Model file for the job. Use its own axes, mm. Face numbers are marked on the shaded views. A direction names the side the tool comes from. Give positions to 0.01 mm unless a question says otherwise; leave off trailing zeros. Write each loop counter-clockwise with the first axis right and the second up, starting at its lowest first coordinate (ties: lowest second). Pieces come first, ordered by that corner, then holes. Notation, with made-up numbers: (61, 57) - (119, 57) arc R22 cw to (119, 90) - close; hole circle Ø8 at (47.25, 0.25). An arc over 180 degrees is marked (long way). Use CSV: the item, a comma, the result in double quotes.
from build123d import *

# Parameters (mm, degrees)
BOSS_EXTRUDE1_DEPTH     = 80
SHELL1_T                = -2
SKETCH2_W               = 15.034493015
SKETCH2_H               = 76
SKETCH2_W_2             = 15.087666062
BOSS_EXTRUDE2_DEPTH     = 2
CUT_EXTRUDE1_REACH      = 82
CUT_EXTRUDE2_REACH      = 82
SKETCH6_R               = 2
CUT_EXTRUDE6_DEPTH      = 61
LPATTERN1_COUNT         = 4
LPATTERN1_PITCH         = 20
MIRROR1_COPY_1_SKETCH_R = 2
MIRROR1_COPY_1_DEPTH    = 61
MIRROR1_COPY_2_SKETCH_R = 2
MIRROR1_COPY_2_DEPTH    = 61
MIRROR1_COPY_3_SKETCH_R = 2
MIRROR1_COPY_3_DEPTH    = 61


with BuildPart() as part:
    # Sketch1 → Boss-Extrude1 (new body)
    with BuildSketch(Plane.XY):
        with BuildLine():
            Line((-75, 0), (75, 0))
            Line((75, 0), (75, 4))
            Line((75, 4), (59.866518188, 4))
            ThreePointArc((59.866518188, 4), (0, 60), (-59.866518188, 4))
            Line((-59.866518188, 4), (-75, 4))
            Line((-75, 4), (-75, 0))
        make_face()
    extrude(amount=BOSS_EXTRUDE1_DEPTH)

    # Shell1
    shell1_openings = [part.faces().sort_by_distance(p)[0] for p in [
        (0, 0, 40),
    ]]
    offset(amount=SHELL1_T, openings=shell1_openings, kind=Kind.INTERSECTION)

    # Sketch2 → Boss-Extrude2 (add)
    with BuildSketch(Plane.XZ.offset(-2)):
        with Locations((-65.482753492, 40)):
            Rectangle(SKETCH2_W, SKETCH2_H)
        with Locations((65.456166969, 40)):
            Rectangle(SKETCH2_W_2, SKETCH2_H)
    extrude(amount=BOSS_EXTRUDE2_DEPTH)

    # Sketch3 → Cut-Extrude1 (cut, up to next)
    with BuildSketch(Plane.XY.offset(80), mode=Mode.PRIVATE) as cut_extrude1_sk1:
        with BuildLine():
            Line((-48.75, 0), (48.75, 0))
            ThreePointArc((48.75, 0), (0, 48.75), (-48.75, 0))
        make_face()
    cut_extrude1_tool1 = extrude(cut_extrude1_sk1.sketch, amount=-CUT_EXTRUDE1_REACH, mode=Mode.PRIVATE) & part.part
    add(cut_extrude1_tool1.solids().sort_by_distance((0, 20.690143, 80))[0], mode=Mode.SUBTRACT)

    # Sketch5 → Cut-Extrude2 (cut, up to next)
    with BuildSketch(Plane(origin=(0, 0, 0), x_dir=(-1, 0, 0), z_dir=(0, 0, -1)), mode=Mode.PRIVATE) as cut_extrude2_sk1:
        with BuildLine():
            Line((-15, 0), (15, 0))
            ThreePointArc((15, 0), (0, 15), (-15, 0))
        make_face()
    cut_extrude2_tool1 = extrude(cut_extrude2_sk1.sketch, amount=-CUT_EXTRUDE2_REACH, mode=Mode.PRIVATE) & part.part
    add(cut_extrude2_tool1.solids().sort_by_distance((0, 6.366198, 0))[0], mode=Mode.SUBTRACT)

    # Sketch6 → Cut-Extrude6 (cut, through all)
    with BuildSketch(Plane.XZ):
        with Locations(Location((67, 70, 0), (0, 0, 270))):  # turned: the seam where the file's is
            Circle(SKETCH6_R)
    cut_extrude6 = extrude(amount=-CUT_EXTRUDE6_DEPTH, mode=Mode.SUBTRACT)

    # LPattern1: Cut-Extrude6 ×4
    with Locations(*[(0, 0, -i * LPATTERN1_PITCH) for i in range(1, LPATTERN1_COUNT)]):
        add(cut_extrude6, mode=Mode.SUBTRACT)

    # Mirror1: Cut-Extrude6 across plane
    add(cut_extrude6.mirror(Plane(origin=(0, 0, 0), x_dir=(0, 0, 1), z_dir=(1, 0, 0))), mode=Mode.SUBTRACT)

    # Mirror1 copy 1 sketch → Mirror1 copy 1 (cut, through all)
    with BuildSketch(Plane(origin=(0, 0, -20), x_dir=(-1, 0, 0), z_dir=(0, -1, 0))):
        with Locations((67, -70)):
            Circle(MIRROR1_COPY_1_SKETCH_R)
    extrude(amount=-MIRROR1_COPY_1_DEPTH, mode=Mode.SUBTRACT)

    # Mirror1 copy 2 sketch → Mirror1 copy 2 (cut, through all)
    with BuildSketch(Plane(origin=(0, 0, -40), x_dir=(-1, 0, 0), z_dir=(0, -1, 0))):
        with Locations((67, -70)):
            Circle(MIRROR1_COPY_2_SKETCH_R)
    extrude(amount=-MIRROR1_COPY_2_DEPTH, mode=Mode.SUBTRACT)

    # Mirror1 copy 3 sketch → Mirror1 copy 3 (cut, through all)
    with BuildSketch(Plane(origin=(0, 0, -60), x_dir=(-1, 0, 0), z_dir=(0, -1, 0))):
        with Locations((67, -70)):
            Circle(MIRROR1_COPY_3_SKETCH_R)
    extrude(amount=-MIRROR1_COPY_3_DEPTH, mode=Mode.SUBTRACT)


solid = part.part
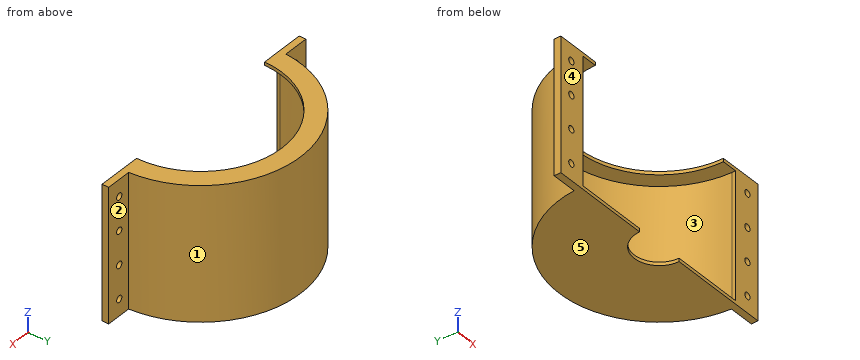
(1) 3-axis set-ups, long thin cutter, end or side, ignore diameter. For the marked faces 1 and 2: which of +Z, -Z, +X, -X, +Y, -Y reach the whole face in a straight line?
Checked values:
face 1,"+Z, -Z, +Y"
face 2,"+Z, -Z, +X, +Y"
(2) Saw through at B-B, the plane x = -67. List the corners of the cut face in (y, z).
Checked values:
outline,"(0, 0) - (4, 0) - (4, 8) - (0, 8) - close; (0, 12) - (4, 12) - (4, 28) - (0, 28) - close; (0, 32) - (4, 32) - (4, 48) - (0, 48) - close; (0, 52) - (4, 52) - (4, 68) - (0, 68) - close; (0, 72) - (4, 72) - (4, 80) - (0, 80) - close"
(3) Wall check: probe 1 along X at (y, z) = (1.3, 10); probe 2 along Z at (x, y) = (27.5, 42); probe 3 along X at (y, z) = (3, 10). Give the ranges that are in metal, low to high. Write a range as [from, to].
Checked values:
probe 1,"x = [-75, -69], [-65, -57.97], [57.91, 65], [69, 75]"
probe 2,"z = [0, 2], [78, 80]"
probe 3,"x = [-75, -69], [-65, -57.92], [57.92, 65], [69, 75]"
(4) Saw through at C-C, the plane y = 12.5. List the corners of the cut face in (x, z), then the cut area to 3 significant figures.
Checked values:
outline,"(-58.68, 0) - (-8.29, 0) - (-8.29, 2) - (-56.64, 2) - (-56.64, 78) - (-47.12, 78) - (-47.12, 80) - (-58.68, 80) - close; (8.29, 0) - (58.68, 0) - (58.68, 80) - (47.12, 80) - (47.12, 78) - (56.64, 78) - (56.64, 2) - (8.29, 2) - close"
area,"559 mm^2"
(5) Pull direction Z, two halves, no side cores. Call the marked faces 3, 4 and 5: released by +Z, released by -Z, zero draft, split by the parting line, or undercut.
Checked values:
face 3,"undercut"
face 4,"zero draft"
face 5,"released by -Z"
(6) Flat gauge pins, fed straight in: P1, Ø2, axis at y = 11.5, z = 69, coming from the +X side; P2, Ø10, axis at y = 16.5, z = 29, coming from the -X side; P3, Ø10, axis at x = -8.5, y = 50.5, coming from the -Z side; P4, Ø2.5, axis at x = -67, z = 50, coming from the -Y side. Where does each tip first touch, or does it go through?
Checked values:
P1,"stops at x = 59.07"
P2,"stops at x = -58.89"
P3,"stops at z = 0"
P4,"passes through"
